Geometry: see drawing. Coordinates: mm, zero at the bounding-box minimum. A direction names the side the tool comes from. Coordinates: 2 decimals unless noted, no trailing zeros. Loops run counter-clockwise (first coordinate to the right, second up) from the corner with the lowest first, then second, coordinate; pieces in that order, holes last. Notation, with made-up numbers: (22.25, 47) -> (28.25, 47) arc R15 ccw to (28.25, 55) -> close; hole circle Ø1 at (-7.5, 79.5). An arc over 180 degrees is marked (long way). Answer as a JSON object with one key per item and string values.
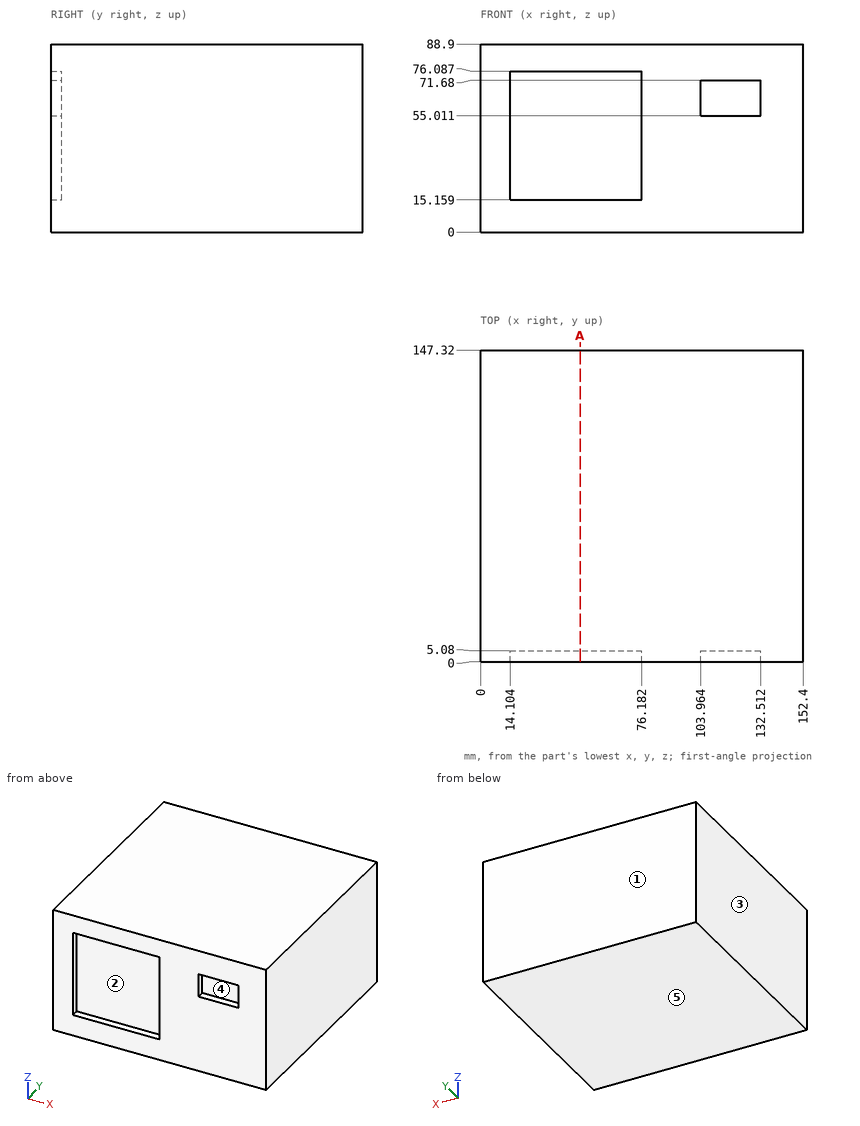
1. Pin query (flat end, axial travel): P1, Ø8, axis at x = 48, y = 18, coming from the -Z side. Return the tip coordinate at first contact, or that it passes through.
Reply:
{"P1": "stops at z = 0"}
2. Line query: line 1 along Y through (x, z) = (36.5, 31). Output: solid intervals per line, ascending.
Reply:
{"line 1": "y = 5.08 to 147.32"}
3. Access query for the marked faces 1 and 2. Directions: +Z, -Z, +X, -X, +Y, -Y. A direction counts if a zero-diameter tool reaches every point of the face in a straight line with its end or side. Return the directions, or none.
Reply:
{"face 1": "+Z, -Z, +X, -X, +Y", "face 2": "-Y"}
4. Mould query, pull axis Z, two halves, no side actions, for the marked faces 3, 4 and 5. Classes: pulls with the +Z half, pulls with the -Z half, needs draft (parallel to the pull), parting line crosses it, or undercut.
Reply:
{"face 3": "needs draft", "face 4": "undercut", "face 5": "pulls with the -Z half"}
5. Section query A-A (x = 47). Return loops of the section in (y, z).
Reply:
{"outline": "(0, 0) -> (147.32, 0) -> (147.32, 88.9) -> (0, 88.9) -> (0, 76.09) -> (5.08, 76.09) -> (5.08, 15.16) -> (0, 15.16) -> close"}
